Here's how the part is built. I have some questions about the finished solid (model axes, mm). A direction names the side the tool comes from. Round coordinates to 2 decimals unless told otherwise and drop trailing zeros. Order: outer loops, then holes, each group sorted by start corner. A loop starts at its lowest first (then second) coordinate and runs counter-clockwise, first axis right, second up.
```python
from build123d import *

# Parameters (mm, degrees)
BOSS_EXTRUDE1_DEPTH     = 50.8
SKETCH2_W               = 81.28
SKETCH2_H               = 50.8
CUT_EXTRUDE1_DEPTH      = 0.254
SKETCH3_R               = 5.3975
CUT_EXTRUDE2_DEPTH      = 6.35
CUT_EXTRUDE3_DEPTH      = 99.778245459
CUT_EXTRUDE3_DEPTH_BACK = 99.778245459
SKETCH4_R               = 3.302
CUT_EXTRUDE4_DEPTH      = 101.578868556
FILLET1_R               = 7.62


with BuildPart() as part:
    # Sketch1 → Boss-Extrude1 (new body)
    with BuildSketch(Plane.XY):
        with BuildLine():
            Line((30.734, 0), (40.64, 0))
            Line((40.64, 0), (40.64, 30.48))
            Line((40.64, 30.48), (0, 30.48))
            Line((0, 30.48), (0, 0))
            Line((0, 0), (11.43, 0))
            ThreePointArc((11.43, 0), (21.082, 9.652), (30.734, 0))
        make_face()
        with BuildLine():
            Line((40.64, 30.48), (40.64, 0))
            Line((40.64, 0), (50.546, 0))
            ThreePointArc((50.546, 0), (60.198, 9.652), (69.85, 0))
            Line((69.85, 0), (81.28, 0))
            Line((81.28, 0), (81.28, 30.48))
            Line((81.28, 30.48), (40.64, 30.48))
        make_face()
    extrude(amount=BOSS_EXTRUDE1_DEPTH)

    # Sketch2 → Cut-Extrude1 (cut)
    with BuildSketch(Plane(origin=(0, 0, 0), x_dir=(-1, 0, 0), z_dir=(0, -1, 0))):
        with Locations((-40.64, -25.4)):
            Rectangle(SKETCH2_W, SKETCH2_H)
    extrude(amount=-CUT_EXTRUDE1_DEPTH, mode=Mode.SUBTRACT)

    # Sketch3 → Cut-Extrude2 (cut)
    with BuildSketch(Plane(origin=(0, 30.48, 0), x_dir=(1, 0, 0), z_dir=(0, 1, 0))):
        with Locations(Location((40.64, -8.89, 0), (0, 0, 270))):
            Circle(SKETCH3_R)
        with Locations(Location((40.64, -41.91, 0), (0, 0, 90))):
            Circle(SKETCH3_R)
        with Locations(Location((40.64, -25.4, 0), (0, 0, 270))):
            Circle(SKETCH3_R)
    extrude(amount=-CUT_EXTRUDE2_DEPTH, mode=Mode.SUBTRACT)

    # Sketch4 → Cut-Extrude3 (cut, two sides: drawn at the far end of the back side and taken through both)
    with BuildSketch(Plane(origin=(0, 24.13, 0), x_dir=(1, 0, 0), z_dir=(0, 1, 0)).offset(-CUT_EXTRUDE3_DEPTH_BACK)):
        with Locations(Location((40.64, -8.89, 0), (0, 0, 270))):
            Circle(SKETCH4_R)
        with Locations(Location((40.64, -41.91, 0), (0, 0, 270))):
            Circle(SKETCH4_R)
        with Locations(Location((40.64, -25.4, 0), (0, 0, 270))):
            Circle(SKETCH4_R)
    extrude(amount=CUT_EXTRUDE3_DEPTH + CUT_EXTRUDE3_DEPTH_BACK, mode=Mode.SUBTRACT)

    # Sketch5 → Cut-Extrude4 (cut, through all)
    with BuildSketch(Plane.XY.offset(50.8)):
        Polygon((7.62, 15.24), (7.62, 25.4), (17.78, 25.4), align=None)
        Polygon((19.576051224, 13.443948776), (19.576051224, 23.603948776), (9.416051224, 13.443948776), align=None)
        Polygon((22.587948776, 23.603948776), (32.747948776, 13.443948776), (22.587948776, 13.443948776), align=None)
        Polygon((24.384, 25.4), (34.544, 15.24), (34.544, 25.4), align=None)
        Polygon((46.736, 15.24), (46.736, 25.4), (56.896, 25.4), align=None)
        Polygon((58.692051224, 13.443948776), (58.692051224, 23.603948776), (48.532051224, 13.443948776), align=None)
        Polygon((61.703948776, 23.603948776), (71.863948776, 13.443948776), (61.703948776, 13.443948776), align=None)
        Polygon((63.5, 25.4), (73.66, 15.24), (73.66, 25.4), align=None)
        Polygon((2.541671342, 2.794), (8.891671342, 2.794), (2.541671342, 9.144), align=None)
        Polygon((3.439696954, 10.042025612), (9.789696954, 3.692025612), (9.789696954, 10.042025612), align=None)
        Polygon((71.490303046, 10.042025612), (77.840303046, 10.042025612), (71.490303046, 3.692025612), align=None)
        Polygon((78.738328658, 9.144), (72.388328658, 2.794), (78.738328658, 2.794), align=None)
    extrude(amount=-CUT_EXTRUDE4_DEPTH, mode=Mode.SUBTRACT)

    # Fillet1
    fillet1_edges = [part.edges().sort_by_distance(p)[0] for p in [
        (0, 30.48, 25.4),
        (81.28, 30.48, 25.4),
    ]]
    fillet(fillet1_edges, radius=FILLET1_R)


solid = part.part
```
1) If we section it at B-B (z = 8.89): Give the number of separate pieces and of enclosed holes in the cut face, plus the area to 3 significant figures.
2) I need wall thicknesses on line 1 (Z direction, x = 40.64, y = 7.5); line 2 (Z direction, x = 40, y = 12); line 3 (Y direction, x = 25.5, z = 7.5). Which ranges of each line are inside material? Lowest first, please.
3) If we section it at C-C (x = 13.5): Write out the boundary of the cut face in (y, z), plus the area to 3 significant figures.
4) I'm going to push flat-ended pins straight in: pin 1 (2 mm diameter, centred on x = 64, y = 6.5, fed in from -Z); pin 2 (3 mm diameter, centred on x = 42.5, z = 27, fed in from +Y); pin 3 (10 mm diameter, centred on x = 58.5, z = 8, fed in from -Y). Where does each tip first touch, or does it pass through?
5) We'd pull the mould along Y, two halves only. Please class faces 4 (the flat face through (6, 0.254, 25)), 5 (the flat face through (41, 24.13, 38)), 6 (the flat face through (30, 25.4, 26)), 7 (the cylindrical face through (35.29, 27.35, 42.61)): +Y half, -Y half, draft (parallel to the pull), parting line (faces both ways), or undercut.
6) If we section it at A-A (x = 40.64): Write out the boundary of the cut face in (y, z).
7) For faces 1 (the cylindrical face through (78.989, 28.307, 25.756)), 2 (the flat face through (13, 25.4, 26)), 3 (the flat face through (38, 24.13, 6)), which set-ups out of +Z, -Z, +X, -X, +Y, -Y let a thin tool reach every point of the face, with its end or its side?
Solutions:
1. separate pieces: 2
1. enclosed holes: 12
1. area: 1,430 mm2
2. line 1: z = 0 to 5.59, 12.19 to 22.1, 28.7 to 38.61, 45.21 to 50.8
2. line 2: z = 0 to 5.65, 12.13 to 22.16, 28.64 to 38.67, 45.15 to 50.8
2. line 3: y = 8.58 to 13.44, 20.69 to 24.28, 25.4 to 30.48
3. outline: (5.97, 0) - (13.44, 0) - (13.44, 50.8) - (5.97, 50.8) - close; (17.53, 0) - (21.12, 0) - (21.12, 50.8) - (17.53, 50.8) - close; (25.4, 0) - (30.48, 0) - (30.48, 50.8) - (25.4, 50.8) - close
3. area: 820 mm2
4. pin 1: passes through
4. pin 2: stops at y = 24.13
4. pin 3: stops at y = 6.95
5. face 4: -Y half
5. face 5: +Y half
5. face 6: undercut
5. face 7: draft
6. outline: (0.25, 0) - (30.48, 0) - (30.48, 3.49) - (24.13, 3.49) - (24.13, 5.59) - (0.25, 5.59) - close; (0.25, 12.19) - (24.13, 12.19) - (24.13, 14.29) - (30.48, 14.29) - (30.48, 20) - (24.13, 20) - (24.13, 22.1) - (0.25, 22.1) - close; (0.25, 28.7) - (24.13, 28.7) - (24.13, 30.8) - (30.48, 30.8) - (30.48, 36.51) - (24.13, 36.51) - (24.13, 38.61) - (0.25, 38.61) - close; (0.25, 45.21) - (24.13, 45.21) - (24.13, 47.31) - (30.48, 47.31) - (30.48, 50.8) - (0.25, 50.8) - close
7. face 1: +Z, -Z, +X, +Y
7. face 2: +Z, -Z
7. face 3: +Y
